Autodesk Inventor part; units mm, degrees
ref_plane "YZ Plane" through (0, 0, 0) normal (1, 0, 0) x (0, 1, 0)
ref_plane "XZ Plane" through (0, 0, 0) normal (0, 1, 0) x (-1, 0, 0)
ref_plane "XY Plane" through (0, 0, 0) normal (0, 0, 1) x (1, 0, 0)
sketch "スケッチ1" plane through (0, 0, 0) normal (1, 0, 0) x (0, 1, 0)
  line L0 (-70, 0) -> (70, 0)
  line L1 (0, 0) -> (0, 4.0415) construction
  line L2 (-69.6874, 4.0415) -> (-70, 3.5)
  line L3 (-70, 3.5) -> (-70, 0)
  line L4 (-69.6874, 4.0415) -> (69.6874, 4.0415)
  line L5 (69.6874, 4.0415) -> (70, 3.5)
  line L6 (70, 3.5) -> (70, 0)
  dimension "d1" = 3.5
  dimension "d2" = 4.0415
  dimension "d3" = 30
  dimension "d4" = 140
revolve "回転1" add sketch "スケッチ1" angle 360 about axis through (0, -70, 0) along (0, 1, 0)
sketch "スケッチ2" plane through (0, 70, 0) normal (0, 1, 0) x (1, 0, 0)
  circle A0 centre (0, 0) radius 4.0415
  line L0 (0, -4.0415) -> (-3.5, -2.0207)
  line L1 (-3.5, -2.0207) -> (-3.5, 2.0207)
  line L2 (-3.5, 2.0207) -> (0, 4.0415)
  line L3 (0, 4.0415) -> (3.5, 2.0207)
  line L4 (3.5, 2.0207) -> (3.5, -2.0207)
  line L5 (3.5, -2.0207) -> (0, -4.0415)
  point P0 (0, 0)
  point P1 (0, 0)
  point P2 (3.5, -2.0207)
  point P3 (3.5, 2.0207)
  point P4 (3.5, 2.0207)
  point P5 (0, 4.0415)
  point P6 (0, 4.0415)
  point P7 (-3.5, 2.0207)
  point P8 (-3.5, 2.0207)
  point P9 (-3.5, -2.0207)
  point P10 (-3.5, -2.0207)
extrude "押し出し1" cut sketch "スケッチ2" against normal through all contours A0 L4 | L3 A0 | A0 L5 | L2 A0 | A0 L0 | L1 A0
hole "穴1" at (0, 70, 0) direction (0, -1, 0) diameter 2.459 depth 6 tip angle 118 countersink diameter 3 countersink angle 90
mirror "ミラー1" about plane through (0, 0, 0) normal (0, 1, 0) of "穴1"
equation "\"d2\" = 1.1547 * d1"
properties part number "ABLSBF7-140-M3-N3" material "アルミニウム 2014-T4"
Here's how the part is built. I have some questions about the finished solid (model axes, mm). A direction names the side the tool comes from. Coordinates: 2 decimals unless noted, no trailing zeros. Write each loop counter-clockwise with the first axis right and the second up, starting at its lowest first coordinate (ties: lowest second). Pieces come first, ordered by that corner, then holes.
1) Which directions (+Z, -Z, +X, -X, +Y, -Y) give clear straight access to the entire face, cutting with the end or side of a thin tool? Please do faces 4 (the face through (-3.5, 1, 0)), 5 (the face through (0.748, 66.825, -0.976)), 6 (the face through (-0.748, -66.825, -0.976)).
Filled in:
face 4: +Z, -Z, -X, +Y, -Y
face 5: +Y
face 6: -Y
2) If I drill on line 1 (Z direction, x = 0, y = 68.5); line 2 (X direction, y = -66.75, z = 0); line 3 (Y direction, x = 2.5, z = 2.5), over which ranges is the centre line in solid material (lowest first)?
Filled in:
line 1: z = -4.04 to -1.23, 1.23 to 4.04
line 2: x = -3.5 to -1.23, 1.23 to 3.5
line 3: y = -69.98 to 69.98
3) If we section it at A-A (y = 61): List the corners of the cut face in (x, z) for me.
Filled in:
outline: (-3.5, -2.02) - (0, -4.04) - (3.5, -2.02) - (3.5, 2.02) - (0, 4.04) - (-3.5, 2.02) - close
4) Thinking about a two-plate mould opening in X: for faces 1 (the face through (0.064, 63.39, 0.204)), 2 (the face through (-0.08, -69.911, 3.653)), 3 (the face through (1.8, 1, 3)), which applies, +X half, -X half, draft (parallel to the pull), parting line (faces both ways), or undercut?
Filled in:
face 1: undercut
face 2: parting line
face 3: +X half
